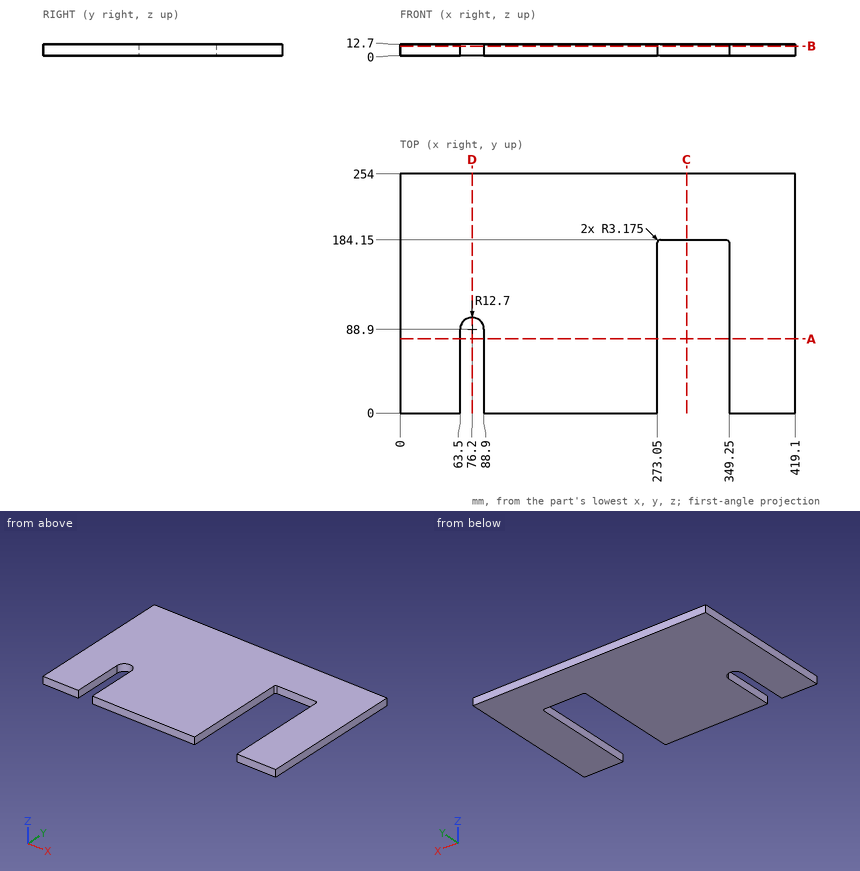
The figure shows three views and two pictorial views of one solid part (mm, origin at its lowest corner). Answer the questions. Give positions to 0.01 mm unless a question says otherwise; leave off trailing zeros. Write each loop counter-clockwise with the first axis right and the second up, starting at its lowest first coordinate (ties: lowest second). Pieces come first, ordered by that corner, then holes. Notation, with made-up numbers: (-28.75, 39.25) - (17.25, 39.25) arc R22 cw to (17.25, 48.25) - close; hole circle Ø5 at (-4.5, 53). An arc over 180 degrees is marked (long way). Use CSV: the item, a comma, the result in double quotes. Start each with the question number.
Item 1: The part is cut by section A-A, the plane y = 79. Give the vertices of the cut face in (x, z).
Item 2: The part is cut by section C-C, the plane x = 304. Give the vertices of the cut face in (y, z), and give its area (3 significant figures).
Item 3: Flat-ended cylindrical pins translate along their axes: P1, Ø1, axis at x = 85, z = 9, coming from the -Y side; P2, Ø5, axis at x = 340, z = 1.5, coming from the -Y side. Find the tip coordinate at first contact, or state that the pin passes through.
Item 4: The part is cut by section D-D, the plane x = 76.2. Give the vertices of the cut face in (y, z), and give its area (3 significant figures).
Item 5: The part is cut by section B-B, the plane z = 10.5. Give the vertices of the cut face in (x, y) (3 decimals).
Item 6: Consider line 1 (X direction, y = 25, z = 2); line 2 (X direction, y = 109, z = 2.5); line 3 (Y direction, x = 346.5, z = 5.5). Determine where each line is inside the solid, lowest interval first.
Taken from the geometry:
1,outline,"(0, 0) - (63.5, 0) - (63.5, 12.7) - (0, 12.7) - close; (88.9, 0) - (273.05, 0) - (273.05, 12.7) - (88.9, 12.7) - close; (349.25, 0) - (419.1, 0) - (419.1, 12.7) - (349.25, 12.7) - close"
2,outline,"(184.15, 0) - (254, 0) - (254, 12.7) - (184.15, 12.7) - close"
2,area,"887 mm2"
3,P1,"y = 97.55"
3,P2,"y = 184.15"
4,outline,"(101.6, 0) - (254, 0) - (254, 12.7) - (101.6, 12.7) - close"
4,area,"1,940 mm2"
5,outline,"(0, 0) - (63.5, 0) - (63.5, 88.9) arc R12.7 cw to (88.9, 88.9) - (88.9, 0) - (273.05, 0) - (273.05, 180.975) arc R3.175 cw to (276.225, 184.15) - (346.075, 184.15) arc R3.175 cw to (349.25, 180.975) - (349.25, 0) - (419.1, 0) - (419.1, 254) - (0, 254) - close"
6,line 1,"0 to 63.5, 88.9 to 273.05, 349.25 to 419.1"
6,line 2,"0 to 273.05, 349.25 to 419.1"
6,line 3,"184.12 to 254"
